Build history of the part. All positions in model axes, mm. A direction names the side the tool comes from. Give positions to 0.01 mm unless a question says otherwise; leave off trailing zeros. Write each loop counter-clockwise with the first axis right and the second up, starting at its lowest first coordinate (ties: lowest second). Pieces come first, ordered by that corner, then holes. Notation, with made-up numbers: (-38, 80) -> (-24, 80) arc R14 ccw to (-24, 104) -> close; hole circle Ø3 at (74, 77.25). An arc over 180 degrees is marked (long way). Write item = value, one per line. Start each with the question number.
Q1. Mould opens along X. For faces 3 (the face through (47, -3, 0)), 4 (the face through (44.37, -13.944, 3.451)), 5 (the face through (94, -3, 2)), 6 (the face through (105, -3, 3)) say: pulls with the +X half, pulls with the -X half, needs draft (parallel to the pull), parting line crosses it, or undercut.
Q2. Saw through at C-C, the plane x = 83. List the corners of the cut face in (y, z), then the cut area to 3 significant figures.
Q3. Wall check: line 1 (Y direction, x = 90, z = 2.5); line 2 (X direction, y = -2, z = 2.25); line 3 (X direction, y = 3.25, z = 4.75). Give the ranges that are in metal, low to high.
Q4. Saw through at D-D, the plane x = 3. List the corners of the cut face in (y, z).
Q5. Saw through at A-A, the plane z = 2.5. List the corners of the cut face in (x, y), then the cut area to 3 significant figures.
Q6. Saw through at B-B, the plane y = -3. List the corners of the cut face in (x, z), then the cut area to 3 significant figures.
Q7. Tool access for faces 1 (the face through (-10, 0, 3)), 2 (the face through (79.96, -2.56, 5.77)): list every direction of +Z, -Z, +X, -X, +Y, -Y with a clear straight run to the whole face (end or side of a thin tool).
Q8. Drop flat-ended pins along their axis: P1, Ø1.5, axis at x = 97, y = -3, coming from the +Z side; P2, Ø2, axis at y = 2, z = 2, coming from the -X side; P3, Ø3, axis at x = 83, y = -3, coming from the +Z side; P4, Ø3, axis at y = -11, z = 1.5, coming from the +X side. Give the stop position or say it passes through.
from build123d import *

# Parameters (mm, degrees)
EXTRUDE_1_DEPTH     = 7
SKETCH_2_R          = 4.1
SKETCH_2_R_2        = 1.25
SKETCH_2_R_3        = 4
CUT_EXTRUDE_1_DEPTH = 10
SKETCH_3_R          = 10.05
CUT_EXTRUDE_2_DEPTH = 2.5
EXTRUDE_START       = -7
SKETCH_4_R          = 4.1
EXTRUDE_5_DEPTH     = 7
SKETCH_6_R          = 4.01
CUT_EXTRUDE_6_DEPTH = 3
SKETCH_8_R          = 1.75
CUT_EXTRUDE_7_DEPTH = 10


with BuildPart() as part:
    # 草图1 → 凸台-拉伸1 (new body)
    with BuildSketch(Plane.XY):
        with BuildLine():
            Line((0, -10), (90, -18))
            ThreePointArc((90, -18), (105, -3), (90, 12))
            Line((90, 12), (0, 10))
            ThreePointArc((0, 10), (-10, 0), (0, -10))
        make_face()
    extrude(amount=EXTRUDE_1_DEPTH)

    # 草图2 → 切除-拉伸1 (cut)
    with BuildSketch(Plane(origin=(0, 0, 0), x_dir=(-1, 0, 0), z_dir=(0, 0, -1))):
        Circle(SKETCH_2_R)
        with Locations((-90, -10)):
            Circle(SKETCH_2_R_2)
        with Locations((-83, -3)):
            Circle(SKETCH_2_R_2)
        with Locations((-90, 4)):
            Circle(SKETCH_2_R_2)
        with Locations((-97, -3)):
            Circle(SKETCH_2_R_2)
        with Locations((-90, -3)):
            Circle(SKETCH_2_R_3)
    extrude(amount=-CUT_EXTRUDE_1_DEPTH, mode=Mode.SUBTRACT)

    # 草图3 → 切除-拉伸2 (cut)
    with BuildSketch(Plane.XY.offset(7)):
        with Locations((90, -3)):
            Circle(SKETCH_3_R)
    extrude(amount=-CUT_EXTRUDE_2_DEPTH, mode=Mode.SUBTRACT)

    # 草图4 → 凸台-拉伸5 (add)
    with BuildSketch(Plane.XY.offset(7).offset(EXTRUDE_START)):
        Circle(SKETCH_4_R)
    extrude(amount=EXTRUDE_5_DEPTH)

    # 草图6 → 切除-拉伸6 (cut)
    with BuildSketch(Plane.XY.offset(7)):
        Circle(SKETCH_6_R)
    extrude(amount=-CUT_EXTRUDE_6_DEPTH, mode=Mode.SUBTRACT)

    # 草图8 → 切除-拉伸7 (cut)
    with BuildSketch(Plane(origin=(0, 0, 0), x_dir=(-1, 0, 0), z_dir=(0, 0, -1))):
        Circle(SKETCH_8_R)
    extrude(amount=-CUT_EXTRUDE_7_DEPTH, mode=Mode.SUBTRACT)


solid = part.part
Report:
q1.face_3 = needs draft
q1.face_4 = pulls with the -X half
q1.face_5 = undercut
q1.face_6 = pulls with the +X half
q2.outline = (-17.38, 0) -> (-4.25, 0) -> (-4.25, 4.5) -> (-10.21, 4.5) -> (-10.21, 7) -> (-17.38, 7) -> close; (-1.75, 0) -> (11.84, 0) -> (11.84, 7) -> (4.21, 7) -> (4.21, 4.5) -> (-1.75, 4.5) -> close
q2.area = 157 mm2
q3.line_1 = -18 to -11.25, -8.75 to -7, 1 to 2.75, 5.25 to 12
q3.line_2 = -9.8 to 82.25, 83.75 to 86.13, 93.87 to 96.25, 97.75 to 104.97
q3.line_3 = -9.46 to -2.35, 2.35 to 82.13, 97.87 to 103.64
q4.outline = (-10.27, 0) -> (10.07, 0) -> (10.07, 7) -> (2.66, 7) -> (2.66, 4) -> (-2.66, 4) -> (-2.66, 7) -> (-10.27, 7) -> close
q5.outline = (0, -10) -> (90, -18) arc R15 ccw to (90, 12) -> (0, 10) arc R10 ccw to start; hole circle Ø3.5 at (0, 0); hole circle Ø2.5 at (83, -3); hole circle Ø8 at (90, -3); hole circle Ø2.5 at (90, -10); hole circle Ø2.5 at (90, 4); hole circle Ø2.5 at (97, -3)
q5.area = 2,680 mm2
q6.outline = (-9.54, 0) -> (81.75, 0) -> (81.75, 4.5) -> (79.95, 4.5) -> (79.95, 7) -> (2.66, 7) -> (2.66, 4) -> (-2.66, 4) -> (-2.66, 7) -> (-9.54, 7) -> close; (84.25, 0) -> (86, 0) -> (86, 4.5) -> (84.25, 4.5) -> close; (94, 0) -> (95.75, 0) -> (95.75, 4.5) -> (94, 4.5) -> close; (98.25, 0) -> (105, 0) -> (105, 7) -> (100.05, 7) -> (100.05, 4.5) -> (98.25, 4.5) -> close
q6.area = 677 mm2
q7.face_1 = +Z, -Z, -X
q7.face_2 = +Z
q8.P1 = through
q8.P2 = -9.95
q8.P3 = 4.5
q8.P4 = 103.52
